Autodesk Inventor part; units mm, degrees
ref_plane "YZ Plane" through (0, 0, 0) normal (1, 0, 0) x (0, 1, 0)
ref_plane "XZ Plane" through (0, 0, 0) normal (0, 1, 0) x (-1, 0, 0)
ref_plane "XY Plane" through (0, 0, 0) normal (0, 0, 1) x (1, 0, 0)
sketch "Sketch1" plane through (0, 0, 0) normal (1, 0, 0) x (0, 1, 0)
  line L0 (0, 0) -> (4, 0)
  line L1 (4, 0) -> (4, -4.5)
  line L2 (4, -4.5) -> (5, -4.5)
  line L3 (5, -4.5) -> (5, -109.3)
  line L4 (5, -109.3) -> (4, -109.3)
  line L5 (4, -109.3) -> (4, -113.8)
  line L6 (4, -113.8) -> (0, -113.8)
  line L7 (0, -113.8) -> (0, 0)
  dimension "d0" = 4.5
  dimension "d1" = 113.8
  dimension "d2" = 5
  dimension "d3" = 4
  dimension "d4" = 4
  dimension "d5" = 4.5
revolve "Revolution1" add sketch "Sketch1" angle 360 about axis through (0, 0, -113.8) along (0, 0, 1)
sketch "Sketch2" plane through (0, 0, 0) normal (1, 0, 0) x (0, 1, 0)
  circle A0 centre (-0.6781, -17.2) radius 3.5
  line L0 (-4, 0) -> (4, 0)
  point P0 (0, 0)
  dimension "d7" = 7
  dimension "d8" = 17.2
extrude "Extrusion1" cut sketch "Sketch2" along normal through all
sketch "Sketch3" plane through (0, 0, 0) normal (1, 0, 0) x (0, 1, 0)
  circle A0 centre (0.378, -38.4) radius 3.5
  line L0 (-4, -113.8) -> (4, -113.8)
  point P0 (0, 0)
  dimension "d11" = 7
  dimension "d12" = 75.4
extrude "Extrusion2" cut sketch "Sketch3" along normal through all
equation "\"d5\" = d0"
properties part number "Mecanum Axle" material "Stainless Steel"
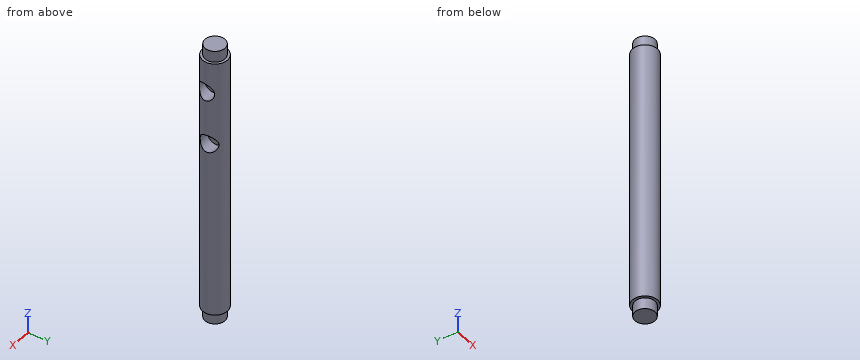
Geometry check sheet. Reference: the model listing, model coordinates, mm. Give positions to 0.01 mm unless a question says otherwise; leave off trailing zeros. Loops run counter-clockwise (first coordinate to the right, second up) from the corner with the lowest first, then second, coordinate; pieces in that order, holes last. Notation, with made-up numbers: M 45,23.5 L 88,23.5 A11 ccw 88,32.5 Z; hole C 20,9.25 d4. An arc over 180 degrees is marked long. Answer as a JSON object with one key per item and string values. Group by question number.
Item 1: Gauge pin test, flat ends, axial feed: pin 1 (5 mm diameter, centred on x = 2, y = 1, fed in from +Z); pin 2 (5 mm diameter, centred on x = 3, z = -81, fed in from +Y); pin 3 (6 mm diameter, centred on y = 3.5, z = -68, fed in from -X); pin 4 (1.5 mm diameter, centred on x = 2.5, z = -56, fed in from +Y). Record the tip position at first contact, or that the pin passes through.
Item 2: Material ranges on L1, parallel to Z at x = 2.75, y = 1.75; L2, parallel to Y at x = 3.15, z = -17.2; L3, parallel to Y at x = 0.25, z = -33.5, recorded low to high.
Item 3: Sectioned sample at D-D on z = -38.4. Record the boundary of the cut face in (x, y).
Item 4: Sectioned sample at A-A on y = 1.75. Record the boundary of the cut face in (x, z), plus the area to 3 significant figures.
Item 5: Sectioned sample at C-C on x = -2.5. Record the boundary of the cut face in (y, z), plus the area to 3 significant figures.
Item 6: Sectioned sample at B-B on z = -79. Record the boundary of the cut face in (x, y).
Findings below:
{
 "1": {"pin 1": "z = 0", "pin 2": "y = 4.97", "pin 3": "x = -4.97", "pin 4": "y = 4.68"},
 "2": {"L1": "-113.8 to -41.62, -35.18 to -19.72, -14.68 to 0", "L2": "2.82 to 3.88", "L3": "-4.99 to 4.99"},
 "3": {"outline": "M 0,-3.12 L 0,3.88 L 3.16,3.88 A5 ccw long 3.91,-3.12 Z"},
 "4": {"outline": "M -4.68,-109.3 L -3.6,-109.3 L -3.6,-113.8 L 3.6,-113.8 L 3.6,-109.3 L 4.68,-109.3 L 4.68,-41.62 L 0,-41.62 L 0,-35.18 L 4.68,-35.18 L 4.68,-19.72 L 0,-19.72 L 0,-14.68 L 4.68,-14.68 L 4.68,-4.5 L 3.6,-4.5 L 3.6,0 L -3.6,0 L -3.6,-4.5 L -4.68,-4.5 Z", "area": "993 mm2"},
 "5": {"outline": "M -4.33,-109.3 L -3.12,-109.3 L -3.12,-113.8 L 3.12,-113.8 L 3.12,-109.3 L 4.33,-109.3 L 4.33,-4.5 L 3.12,-4.5 L 3.12,0 L -3.12,0 L -3.12,-4.5 L -4.33,-4.5 Z", "area": "964 mm2"},
 "6": {"outline": "C 0,0 d10"}
}
